Could you check a few things on this model? Use its own coordinates, in mm. A direction names the side the tool comes from. Coordinates: 2 decimals unless noted, no trailing zeros. Loops run counter-clockwise (first coordinate to the right, second up) from the corner with the lowest first, then second, coordinate; pieces in that order, holes last. Notation, with made-up numbers: M -10,54 L -2,54 A22 ccw -2,90 Z; hole C 16,32.5 d5. An arc over 180 degrees is marked long. Use one line per item in the form item = value. Start each with the question number.
```python
from build123d import *

# Parameters (mm, degrees)
SKETCH7_R           = 10.735
BASE_FLANGE1_DEPTH  = 1
SKETCH17_R          = 4
SKETCH17_R_2        = 2.5
BOSS_EXTRUDE1_DEPTH = 4


# Read off the part's stored shape, not the designer's step: Edge-Flange1
# Sheet-metal steps are written as plain solids
with BuildPart() as part:
    # Sketch7 → Base-Flange1 (new body)
    with BuildSketch(Plane(origin=(0, 0, 0), x_dir=(1, 0, 0), z_dir=(0, 1, 0))):
        with Locations(Location((0, 0, 0), (0, 0, 270))):
            Circle(SKETCH7_R)
    extrude(amount=-BASE_FLANGE1_DEPTH)

    # Edge-Flange1 outline → Edge-Flange1 (revolve, cut)
    with BuildSketch(Plane.XY):
        with BuildLine():
            Line((10.57104109, -1), (10.735, -1))
            Line((10.735, -1), (10.735, 0))
            Line((10.735, 0), (8.9984, 0))
            ThreePointArc((8.9984, 0), (9.930226164, -0.271171885), (10.57104109, -1))
        make_face()
    revolve(axis=Axis((0, 0, 0), (0, 1, 0)), mode=Mode.SUBTRACT)

    # Edge-Flange1 2 outline → Edge-Flange1 2 (revolve)
    with BuildSketch(Plane.XY):
        with BuildLine():
            Line((9.735, -1.7366), (9.735, -15))
            Line((9.735, -15), (10.735, -15))
            Line((10.735, -15), (10.735, -1.7366))
            ThreePointArc((10.735, -1.7366), (10.693514757, -1.359286442), (10.57104109, -1))
            Line((10.57104109, -1), (8.9984, -1))
            ThreePointArc((8.9984, -1), (9.519254855, -1.215745145), (9.735, -1.7366))
        make_face()
    revolve(axis=Axis((0, 0, 0), (0, 1, 0)))

    # Sketch17 → Boss-Extrude1 (add)
    with BuildSketch(Plane.XZ.offset(1)):
        with Locations(Location((0, 0, 0), (0, 0, 90))):
            Circle(SKETCH17_R)
        with Locations(Location((0, 0, 0), (0, 0, 270))):
            Circle(SKETCH17_R_2, mode=Mode.SUBTRACT)
    extrude(amount=BOSS_EXTRUDE1_DEPTH)


solid = part.part
```
Item 1: I'm going to push flat-ended pins straight in: P1, Ø5, axis at y = -2.5, z = 8, coming from the -X side; P2, Ø5.5, axis at x = 1, z = -2.5, coming from the -Y side; P3, Ø8, axis at x = 0, z = 0, coming from the +Y side; P4, Ø1, axis at y = -7, z = -7.5, coming from the -X side. Where does each tip first touch, or does it pass through?
Item 2: Please list where these lines run through material, in increasing order: line 1 along X through (y, z) = (-3.7, 0) (3 decimals); line 2 along Z through (x, y) = (0, -10) (3 decimals); line 3 along Z through (x, y) = (-1.5, -3.25).
Item 3: For faces 1 (the cylindrical face through (9.285, -8.461, -2.924)), 2 (the flat face through (-5, -15, 9)), which set-ups out of +Z, -Z, +X, -X, +Y, -Y let a thin tool reach every point of the face, with its end or its side?
Item 4: Thinking about a two-plate mould opening in X: for faces 3 (the flat face through (-2, -1, 4)), 4 (the flat face through (-2, -5, 2)), 5 (the cylindrical face through (10.24, -8.28, -3.22)), 6 (the flat face through (0, 0, 0)), which applies, pulls with the +X half, pulls with the -X half, needs draft (parallel to the pull), parting line crosses it, or undercut?
Item 5: I want a section at A-A (y = -5.5). Write out the boundary of the cut face in (x, z) (3 decimals).
Worked answers:
q1.P1 = -9.22
q1.P2 = -5
q1.P3 = 0
q1.P4 = -8.14
q2.line_1 = -10.735 to -9.735, -4 to -2.5, 2.5 to 4, 9.735 to 10.735
q2.line_2 = -10.735 to -9.735, 9.735 to 10.735
q2.line_3 = -10.63 to -9.62, -3.71 to -2, 2 to 3.71, 9.62 to 10.63
q3.face_1 = -Y
q3.face_2 = +Z, -Z, +X, -X, -Y
q4.face_3 = undercut
q4.face_4 = undercut
q4.face_5 = parting line crosses it
q4.face_6 = needs draft
q5.outline = C 0,0 d21.47; hole C 0,0 d19.47
